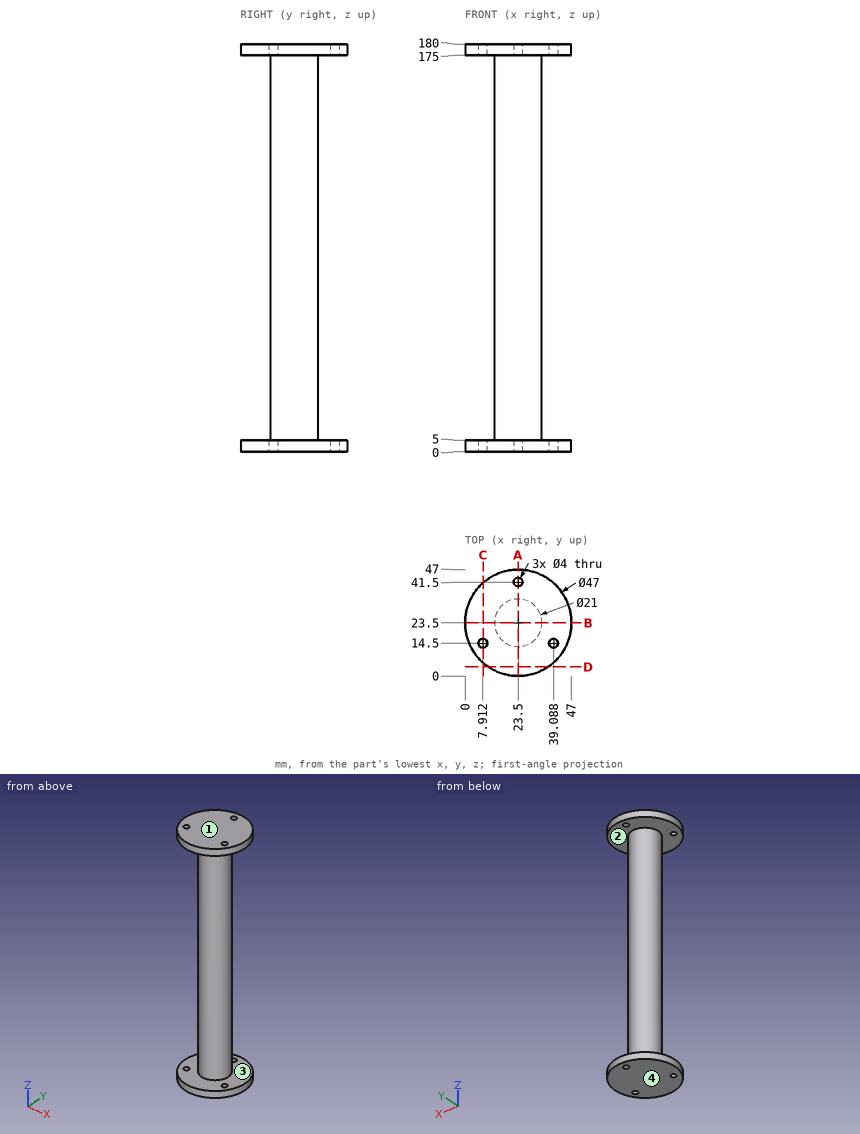
Geometry: see drawing. Coordinates: mm, zero at the bounding-box minimum. Round coordinates to 2 decimals unless told otherwise and drop trailing zeros. Order: outer loops, then holes, each group sorted by start corner. A loop starts at its lowest first (then second) coordinate and runs counter-clockwise, first axis right, second up. Notation, with made-up numbers: (59.5, 42) - (88.5, 42) arc R15 cw to (88.5, 54) - close; hole circle Ø11 at (2, -39). An arc over 180 degrees is marked (long way). Use a Markdown table: item, result. Add a question column.
1. Mould query, pull axis Z, two halves, no side actions, for the marked faces 1, 2, 3 and 4. Classes: +Z half, -Z half, draft (parallel to the pull), parting line (faces both ways), or undercut.
2. Line query: probe 1 along Z at (x, y) = (24, 45.5); probe 2 along X at (y, z) = (14, 3) (1 decimal); probe 3 along X at (y, z) = (41, 2) (1 decimal). Output: solid intervals per line, ascending.
3. Section query D-D (y = 4). Return the cut outline in (x, z) (1 decimal).
4. Section query C-C (x = 8). Return the cut outline in (y, z), then the cut area to 3 significant figures.
5. Section query A-A (x = 23.5). Return the cut outline in (y, z).
6. First-contact query: pin 1 (5 mm diameter, centred on x = 7.91, y = 14.5, fed in from -Z); pin 2 (8 mm diameter, centred on y = 10.5, z = 99.5, fed in from -X); pin 3 (1.5 mm diameter, centred on x = 17.5, z = 109, fed in from -Y); pin 4 (1 mm diameter, centred on x = 32, z = 40.5, fed in from +Y). Flat tips, straight axial feed; report the tip coordinate or a pass-through.
7. Section query B-B (y = 23.5). Return the cut outline in (x, z).
Derived:
| question | item | result |
|---|---|---|
| 1 | face 1 | +Z half |
| 1 | face 2 | undercut |
| 1 | face 3 | undercut |
| 1 | face 4 | -Z half |
| 2 | probe 1 | 0 to 5, 175 to 180 |
| 2 | probe 2 | 2 to 6, 9.8 to 37.2, 41 to 45 |
| 2 | probe 3 | 7.8 to 21.6, 25.4 to 39.2 |
| 3 | outline | (10.4, 0) - (36.6, 0) - (36.6, 5) - (10.4, 5) - close; (10.4, 175) - (36.6, 175) - (36.6, 180) - (10.4, 180) - close |
| 4 | outline | (5.84, 0) - (12.5, 0) - (12.5, 5) - (5.84, 5) - close; (5.84, 175) - (12.5, 175) - (12.5, 180) - (5.84, 180) - close; (16.5, 0) - (41.16, 0) - (41.16, 5) - (16.5, 5) - close; (16.5, 175) - (41.16, 175) - (41.16, 180) - (16.5, 180) - close |
| 4 | area | 313 mm2 |
| 5 | outline | (0, 0) - (39.5, 0) - (39.5, 5) - (34, 5) - (34, 175) - (39.5, 175) - (39.5, 180) - (0, 180) - (0, 175) - (13, 175) - (13, 5) - (0, 5) - close; (43.5, 0) - (47, 0) - (47, 5) - (43.5, 5) - close; (43.5, 175) - (47, 175) - (47, 180) - (43.5, 180) - close |
| 6 | pin 1 | z = 0 |
| 6 | pin 2 | x = 18.09 |
| 6 | pin 3 | y = 14.41 |
| 6 | pin 4 | y = 30.3 |
| 7 | outline | (0, 0) - (47, 0) - (47, 5) - (34, 5) - (34, 175) - (47, 175) - (47, 180) - (0, 180) - (0, 175) - (13, 175) - (13, 5) - (0, 5) - close |
